from build123d import *

# Parameters (mm, degrees)
SKETCH2_W                = 15
SKETCH2_H                = 20
BOSS_EXTRUDE1_DEPTH      = 50
BOSS_EXTRUDE1_DEPTH_BACK = 50
CUT_EXTRUDE1_DEPTH       = 8.5
FILLET1_R                = 0.302678334
LPATTERN1_COUNT          = 21
LPATTERN1_PITCH          = 4.7124
FILLET1_OF_LPATTERN1_R   = 0.302678334


with BuildPart() as part:
    # Sketch2 → Boss-Extrude1 (new body, two sides)
    with BuildSketch(Plane(origin=(0, 0, 0), x_dir=(0, 0, -1), z_dir=(1, 0, 0))) as boss_extrude1_sk:
        with Locations((0, 10)):
            Rectangle(SKETCH2_W, SKETCH2_H)
    extrude(amount=BOSS_EXTRUDE1_DEPTH)
    extrude(boss_extrude1_sk.sketch, amount=-BOSS_EXTRUDE1_DEPTH_BACK)

    # Sketch3 → Cut-Extrude1 (cut, symmetric)
    with BuildSketch(Plane.XY):
        Polygon((-48.735710703, 20), (-47.516119242, 16.6492), (-46.507191461, 16.6492), (-45.2876, 20), align=None)
    cut_extrude1 = extrude(amount=CUT_EXTRUDE1_DEPTH, both=True, mode=Mode.SUBTRACT)

    # Fillet1
    fillet1_edges = [part.edges().sort_by_distance(p)[0] for p in [
        (-46.507191461, 16.6492, 0),
        (-47.516119242, 16.6492, 0),
    ]]
    fillet(fillet1_edges, radius=FILLET1_R)

    # LPattern1: Cut-Extrude1 ×21
    with Locations(*[(i * LPATTERN1_PITCH, 0, 0) for i in range(1, LPATTERN1_COUNT)]):
        add(cut_extrude1, mode=Mode.SUBTRACT)

    # Fillet1 of LPattern1
    fillet1_of_lpattern1_edges = [part.edges().sort_by_distance(p)[0] for p in [
        (-41.794791461, 16.6492, 0),
        (-42.803719242, 16.6492, 0),
        (-37.082391461, 16.6492, 0),
        (-38.091319242, 16.6492, 0),
        (-32.369991461, 16.6492, 0),
        (-33.378919242, 16.6492, 0),
        (-27.657591461, 16.6492, 0),
        (-28.666519242, 16.6492, 0),
        (-22.945191461, 16.6492, 0),
        (-23.954119242, 16.6492, 0),
        (-18.232791461, 16.6492, 0),
        (-19.241719242, 16.6492, 0),
        (-13.520391461, 16.6492, 0),
        (-14.529319242, 16.6492, 0),
        (-8.807991461, 16.6492, 0),
        (-9.816919242, 16.6492, 0),
        (-4.095591461, 16.6492, 0),
        (-5.104519242, 16.6492, 0),
        (0.616808539, 16.6492, 0),
        (-0.392119242, 16.6492, 0),
        (5.329208539, 16.6492, 0),
        (4.320280758, 16.6492, 0),
        (10.041608539, 16.6492, 0),
        (9.032680758, 16.6492, 0),
        (14.754008539, 16.6492, 0),
        (13.745080758, 16.6492, 0),
        (19.466408539, 16.6492, 0),
        (18.457480758, 16.6492, 0),
        (24.178808539, 16.6492, 0),
        (23.169880758, 16.6492, 0),
        (28.891208539, 16.6492, 0),
        (27.882280758, 16.6492, 0),
        (33.603608539, 16.6492, 0),
        (32.594680758, 16.6492, 0),
        (38.316008539, 16.6492, 0),
        (37.307080758, 16.6492, 0),
        (43.028408539, 16.6492, 0),
        (42.019480758, 16.6492, 0),
        (47.740808539, 16.6492, 0),
        (46.731880758, 16.6492, 0),
    ]]
    fillet(fillet1_of_lpattern1_edges, radius=FILLET1_OF_LPATTERN1_R)


solid = part.part
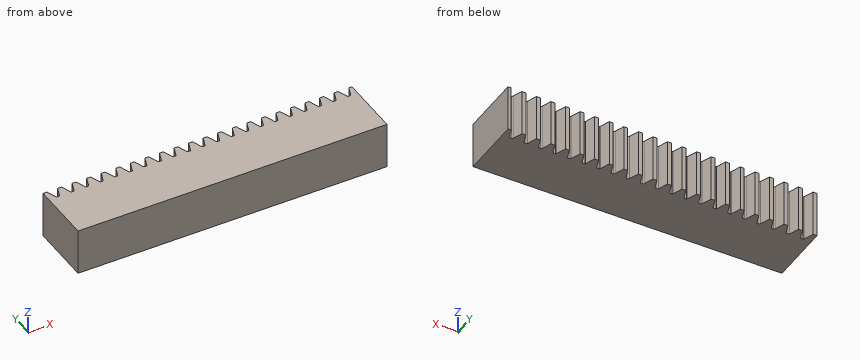
Check sheet for the modelled part. Datum: model origin and axes. Units: mm. Round coordinates to 2 decimals unless told otherwise and drop trailing zeros. Return JSON: item names as keys, results as strings.
Q1. Depth check by flat-ended pin: P1, Ø0.5, axis at x = -47, z = -0.5, coming from the +Y side; P2, Ø0.5, axis at x = 0, z = -2, coming from the +Y side. Enter the tip coordinate at first touch or a pass-through.
Returned:
{"P1": "stops at y = 16.65", "P2": "stops at y = 16.66"}
Q2. Cross-section at A-A (y = 19). Give the number of separate pieces and of enclosed holes in the cut face, then the cut area to 3 significant figures.
Returned:
{"separate pieces": "22", "enclosed holes": "0", "area": "643 mm²"}
Q3. Scan line: L1, parallel to Y at x = 42, z = 3. Record every from-to range of solid material in increasing order. Write a range as from..to.
Returned:
{"L1": "y = 0..16.76"}
